The model under review builds one solid part; all positions refer to its coordinate system, in mm. A direction names the side the tool comes from. Round coordinates to 2 decimals unless told otherwise and drop trailing zeros. Write each loop counter-clockwise with the first axis right and the second up, starting at its lowest first coordinate (ties: lowest second). Pieces come first, ordered by that corner, then holes. Notation, with made-up numbers: M 19,-25.75 L 70,-25.75 A20 cw 70,-5.75 Z; hole C -10.5,15 d2. An arc over 180 degrees is marked long. Write item = value, one per line. Start each with the question number.
Item 1: Tool access review of faces 1 (the flat face through (13, -22, 90)), 2 (the flat face through (6, -22, 89.049)): name each direction out of +Z, -Z, +X, -X, +Y, -Y from which nothing blocks a thin tool from reaching the whole face with its end or side.
Item 2: Take a section at A-A, the plane z = 56.5. Give the boundary of the cut face in (x, y), plus the area to 3 significant figures.
Item 3: For pin 1 Ø2 at (x, y) = (6.5, -25) entering from -Z; pin 2 Ø1 at (y, z) = (-9.5, 91.5) entering from -X, all flat-tipped, find the tip position at first contact; note any pin that passes through.
Item 4: Take a section at B-B, the plane x = 6. Give the boundary of the cut face in (y, z), plus the area to 3 significant figures.
Item 5: To check wall thickness, follow line 1 along Y through (x, z) = (3.25, 50); line 2 along Z through (x, y) = (3.25, -3). State the ranges of each line that lie inside material, in increasing order.
Item 6: The part is to be moulded in two halves that separate along Y. For faces 3 (the flat face through (6, 0, 57)), 4 (the flat face through (6, -45.288, 58)), 5 (the flat face through (6, -55.288, 63)), 6 (the flat face through (6, 5, 25.4)), say which applies: +Y half, -Y half, draft (parallel to the pull), parting line (faces both ways), or undercut.
Item 7: Take a section at C-C, the plane y = -16. Give the boundary of the cut face in (x, z), plus the area to 3 significant figures.
Autodesk Fusion 360 part; units mm, degrees
sketch "Sketch1" plane through (0, 0, 0) normal (1, 0, 0) x (0, 0, -1)
  line L0 (-25.4, 25.4) -> (25.4, 25.4)
  line L1 (25.4, 25.4) -> (25.4, -63.5)
  line L2 (25.4, -63.5) -> (-25.4, -63.5)
  line L3 (-25.4, -63.5) -> (-25.4, 25.4)
sketch "Sketch2" plane through (0, 0, 0) normal (1, 0, 0) x (0, 0, -1)
  line L0 (0, 0) -> (-89.049, 0)
  line L1 (-89.049, 0) -> (-89.049, -45.288)
  line L2 (-89.049, -45.288) -> (0, -45.288)
  line L3 (0, -45.288) -> (0, 0)
  line L4 (10, 10) -> (-99.049, 10)
  line L5 (-99.049, 10) -> (-99.049, -55.288)
  line L6 (-99.049, -55.288) -> (10, -55.288)
  line L7 (10, -55.288) -> (10, 10)
  line L8 (-25.4, -63.5) -> (-25.4, 25.4)
  dimension "d1" = 89.049
  dimension "d2" = 45.288
  dimension "d3" = 109.049
  dimension "d4" = 65.288
  dimension "d6" = 10
  dimension "d7" = 10
  dimension "d8" = 25.4
extrude "Extrude1" add sketch "Sketch2" along normal blind 13 contours L0 L2 L3 L4 L6 L7 L8 | L0 L1 L2 L4 L5 L6 L8
extrude "Extrude2" cut sketch "Sketch1" along normal blind 13
sketch "Sketch3" plane through (0, 0, 0) normal (1, 0, 0) x (0, 0, -1)
Response values:
q1.face_1 = +Z, -Z, +X, +Y, -Y
q1.face_2 = -Z, +X, -X
q2.outline = M 0,-55.29 L 13,-55.29 L 13,-45.29 L 0,-45.29 Z; M 0,0 L 13,0 L 13,10 L 0,10 Z
q2.area = 260 mm2
q3.pin_1 = 89.05
q3.pin_2 = 0
q4.outline = M -55.29,25.4 L -45.29,25.4 L -45.29,89.05 L 0,89.05 L 0,25.4 L 10,25.4 L 10,99.05 L -55.29,99.05 Z
q4.area = 1,930 mm2
q5.line_1 = -55.29 to -45.29, 0 to 10
q5.line_2 = 89.05 to 99.05
q6.face_3 = undercut
q6.face_4 = undercut
q6.face_5 = -Y half
q6.face_6 = draft
q7.outline = M 0,89.05 L 13,89.05 L 13,99.05 L 0,99.05 Z
q7.area = 130 mm2
